Model file for the job. Use its own axes, mm. A direction names the side the tool comes from. Coordinates: 2 decimals unless noted, no trailing zeros. Order: outer loops, then holes, each group sorted by start corner. A loop starts at its lowest first (then second) coordinate and runs counter-clockwise, first axis right, second up. Notation, with made-up numbers: M 69,77.5 L 110,77.5 A28 cw 110,100.5 Z; hole C 79,-2.75 d10. An arc over 180 degrees is marked long. Return JSON: item names as keys, results as strings.
Autodesk Inventor part; units mm, degrees
ref_plane "Work Plane1" through (-56, -20.6155, 4) normal (0, 0, -1) x (-1, 0, 0)
ref_plane "YZ Plane" through (0, 0, 0) normal (1, 0, 0) x (0, 1, 0)
ref_plane "XZ Plane" through (0, 0, 0) normal (0, 1, 0) x (-1, 0, 0)
sketch "Sketch1" plane through (0, 0, 0) normal (0, 0, 1) x (1, 0, 0)
  line L0 (0, -4.2) -> (0, 25.2) construction
  line L1 (-78.4, 0) -> (78.4, 0) construction
  line L2 (-45, 16) -> (45, 16)
  line L3 (45, 16) -> (45, 0)
  line L4 (45, 0) -> (-45, 0)
  line L5 (-45, 0) -> (-45, 16)
  line L6 (-45, 0) -> (-51, 0)
  line L7 (-51, 0) -> (-51, 21)
  line L8 (-51, 21) -> (-45, 16)
  line L9 (-51, 21) -> (-56, 21)
  line L10 (-56, 21) -> (-56, 0)
  line L11 (-56, 0) -> (-51, 0)
  line L12 (-51, 0) -> (-51, 21)
  line L13 (45, 0) -> (45, 16)
  line L14 (45, 0) -> (51, 0)
  line L15 (51, 0) -> (51, 21)
  line L16 (51, 21) -> (45, 16)
  line L17 (51, 21) -> (56, 21)
  line L18 (56, 21) -> (56, 0)
  line L19 (56, 0) -> (51, 0)
  line L20 (51, 0) -> (51, 21)
  point P0 (0, 0)
  dimension "d1" = 90
  dimension "d3" = 6
  dimension "d4" = 5
  dimension "d6" = 5
  dimension "d7" = 16
  dimension "d9" = 11
revolve "Revolution1" add sketch "Sketch1" angle 360 about axis through (-10, 0, 0) along (1, 0, 0)
sketch "Sketch2" plane through (-56, 0, 0) normal (-1, 0, 0) x (0, 0, 1)
  line L0 (-30.6, 0) -> (29.6, 0) construction
  line L1 (-4, 20.6155) -> (-21, 20.6155)
  line L2 (-21, 20.6155) -> (-21, -20.6155)
  line L3 (-21, -20.6155) -> (-4, -20.6155)
  line L4 (-4, -20.6155) -> (-4, 20.6155)
  circle A0 centre (0, 0) radius 16 construction
  circle A1 centre (0, 0) radius 16 construction
  circle A2 centre (0, 0) radius 16 construction
  line L5 (0, 0) -> (16, 0) construction
  circle A3 centre (0, 0) radius 16 construction
  circle A4 centre (0, 0) radius 21 construction
  dimension "d8" = 20
extrude "Extrusion1" cut sketch "Sketch2" against normal blind 59.25
sketch "Sketch3" plane through (-56, -20.6155, -4) normal (0, 0, -1) x (-1, 0, 0)
  line L0 (0, 41.6155) -> (0, -0.3845) construction
  line L1 (0, 20.6155) -> (-59.25, 20.6155) construction
  line L2 (-59.25, 36.1075) -> (-59.25, 5.1236) construction
  circle A0 centre (-41.25, 20.6155) radius 2.15
  circle A1 centre (-51.25, 20.6155) radius 2.15
  line L3 (-41.25, 20.6155) -> (-51.25, 20.6155) construction
  line L4 (-11, 36.6155) -> (-11, 4.6155) construction
  line L5 (-11, 4.6155) -> (-11, 36.6155) construction
  line L6 (-5, 41.6155) -> (-11, 36.6155) construction
  line L7 (-11, 5.1236) -> (-59.25, 5.1236) construction
  line L8 (-56.25, 5.1236) -> (-56.25, 36.1075) construction
  line L9 (-59.25, 36.1075) -> (-11, 36.1075) construction
  point P0 (-56, 20.6155)
  point P1 (0, 41.2311)
  point P2 (0, 0)
  point P3 (-46.25, 20.6155)
  dimension "d14" = 4.3
  dimension "d16" = 10
  dimension "d18" = 4.3
  dimension "d21" = 3
  dimension "d22" = 10
extrude "Extrusion2" cut sketch "Sketch3" against normal up to surface
ref_plane "Work Plane1" through (-56, -20.6155, 4) normal (0, 0, -1) x (-1, 0, 0)
sketch "Sketch4" plane through (-56, -20.6155, 4) normal (0, 0, -1) x (-1, 0, 0)
  circle A0 centre (-41.25, 20.6155) radius 2.15
  circle A1 centre (-41.25, 20.6155) radius 4
  circle A2 centre (-51.25, 20.6155) radius 2.15
  circle A3 centre (-51.25, 20.6155) radius 4
  point P0 (-56, 20.6155)
  dimension "d24" = 8
  dimension "d25" = 8
extrude "Extrusion3" cut sketch "Sketch4" against normal up to surface contours A0 | A1 | A2 | A3
chamfer "Chamfer1" distance 3 angle 45 1 edges at (56, -21, 0)
equation "\"d8\" = ShaftH"
equation "\"d10\" = d92 + d9 + LCClearance"
equation "\"d21\" = LCClearance"
equation "\"d26\" = d92 + d9 + LCClearance"
equation "\"ShaftH\" = 20"
equation "\"WallT\" = 3"
equation "\"SpoolOffset\" = 8"
equation "\"BottomT\" = 4"
equation "\"WallH\" = 45"
equation "\"ShaftL\" = 81"
equation "\"LCClearance\" = 3"
properties part number "FS_ShaftV2"
Item 1: Saw through at B-B (x = -4.75). Write the cut outline in (y, z).
Check result:
{"outline": "M -15.49,-4 L -2.15,-4 L -2.15,4 L -4,4 L -4,15.49 A16 ccw Z; M 2.15,-4 L 15.49,-4 A16 ccw 4,15.49 L 4,4 L 2.15,4 Z"}
Item 2: Pull direction X, two halves, no side cores. Call faces 1 (the cylindrical face through (-10.754, 0.176, 9.916)), 2 (the conical face through (55.81, -3.94, 17.76)), 3 (the flat face through (3.25, 0, -9)): +X half, -X half, draft (parallel to the pull), parting line (faces both ways), or undercut.
Check result:
{"face 1": "undercut", "face 2": "+X half", "face 3": "-X half"}
Item 3: 3-axis set-ups, long thin cutter, end or side, ignore diameter. For faces 4 (the flat face through (-6, -2, 4)), 5 (the flat face through (-27, 0, -4)), 6 (the cylindrical face through (10.63, -2.083, 15.864)), 7 (the cylindrical face through (-16.8, 0.65, -0.06)): which of +Z, -Z, +X, -X, +Y, -Y reach the whole face in a straight line?
Check result:
{"face 4": "+Z", "face 5": "-Z, -X, +Y, -Y", "face 6": "none", "face 7": "+Z, -Z"}
Item 4: Saw through at C-C (z = 0). Write the cut outline in (x, y), and give its area (3 significant figures).
Check result:
{"outline": "M -56,-21 L -51,-21 L -45,-16 L 45,-16 L 51,-21 L 53,-21 L 56,-18 L 56,18 L 53,21 L 51,21 L 45,16 L -45,16 L -51,21 L -56,21 Z; hole C -14.75,0 d4.3; hole C -4.75,0 d4.3", "area": "3,710 mm2"}
Item 5: Drop flat-ended pins along their axis: pin 1 Ø10 at (x, y) = (32, -1.5) entering from +Z; pin 2 Ø6 at (x, y) = (10, 6.5) entering from -Z; pin 3 Ø2.5 at (x, y) = (-14, -1.5) entering from +Z; pin 4 Ø2.5 at (x, y) = (-4.75, 0) entering from -Z. Give the stop position or say it passes through.
Check result:
{"pin 1": "stops at z = 16", "pin 2": "stops at z = -15.61", "pin 3": "stops at z = 4", "pin 4": "passes through"}
Item 6: Saw through at A-A (y = 0). Count the separate pieces of the cut face and the enclosed holes in it, and give its area (3 significant figures).
Check result:
{"separate pieces": "3", "enclosed holes": "0", "area": "2,720 mm2"}
Item 7: Saw through at D-D (x = 48). Write the cut outline in (y, z), and give its area (3 significant figures).
Check result:
{"outline": "C 0,0 d37", "area": "1,080 mm2"}
Item 8: Wall check: line 1 (X direction, y = 0, z = 9.25); line 2 (X direction, y = -3, z = 6); line 3 (Y direction, x = -4.75, z = -0.75). Give the ranges that are in metal, low to high.
Check result:
{"line 1": "x = -56 to -18.75, -10.75 to -8.75, -0.75 to 56", "line 2": "x = -56 to -17.4, -12.1 to -7.4, -2.1 to 56", "line 3": "y = -15.98 to -2.15, 2.15 to 15.98"}
